Geometry: final body of the model. Coordinates: model frame, mm. A direction names the side the tool comes from. Round coordinates to 2 decimals unless told otherwise and drop trailing zeros. Loops run counter-clockwise (first coordinate to the right, second up) from the corner with the lowest first, then second, coordinate; pieces in that order, holes last. Notation, with made-up numbers: (53, 89) - (93, 89) arc R20 cw to (93, 121) - close; hole circle Ø3 at (0.25, 34.25). An arc over 180 degrees is marked (long way). Return JSON: item names as keys, results as strings. Group by question number.
1. Section A-A on x = 27. Return loops of the section in (y, z), and give its area (3 significant figures).
2. Set-up query: faces 4 (the face through (23.47, -16.04, 4.93)), 5 (the face through (-0.27, -19.57, 4.99)), 6 (the face through (0, 26, 6)), 7 (the face through (-6, -9, 10)), 8 (the face through (2.1, -7.072, 3.8)). Return all of +Z, -Z, +X, -X, +Y, -Y with unobstructed straight access to the full face (end or side cutting, diameter ignored); none if empty.
3. Draft query along Z for faces 1 (the face through (0, -12, 6)), 2 (the face through (28.79, -10.06, 4.93)), 3 (the face through (-6, -9, 0)). Return one class per face: +Z half, -Z half, draft (parallel to the pull), parting line (faces both ways), or undercut.
4. Section D-D on y = 27.5. Return loops of the section in (x, z).
5. Section C-C on z = 3. Return loops of the section in (x, y), and give its area (3 significant figures).
6. First-contact query: pin 1 Ø1 at (y, z) = (22, 3.5) entering from -X; pin 2 Ø6 at (x, z) = (0.5, 3.5) entering from -Y; pin 3 Ø1 at (x, z) = (14, 5.5) entering from -Y; pin 4 Ø2 at (x, z) = (11, 2.5) entering from +Y. Flat tips, straight axial feed; report the tip coordinate or a pass-through.
7. Material intervals for probe 1 along Z at (x, y) = (9.5, -8.5); probe 2 along Y at (x, z) = (8, 9.5); probe 3 along Y at (x, z) = (-14, 2.5), sorted ascending.
8. Section B-B on x = 0. Return loops of the section in (y, z).
from build123d import *

# Parameters (mm, degrees)
F1_DEPTH = 10
F2_DEPTH = 6
F3_DEPTH = 10
F4_START = 4
F4_DEPTH = 2


with BuildPart() as f1:
    # F0 (on Top) → F1 (new body)
    with BuildSketch(Plane.XY):
        with BuildLine():
            ThreePointArc((-28.7731093646, 19.9275732966), (0, 35), (28.7731093646, 19.9275732966))
            Line((28.7731093646, 19.9275732966), (31.0875692673, 22.4657579282))
            ThreePointArc((31.0875692673, 22.4657579282), (32.4897132735, 26.1572999971), (30.9896112585, 29.8101324057))
            ThreePointArc((30.9896112585, 29.8101324057), (-42.9603623337, 1.8458786953), (28.3184138379, -32.358421434))
            ThreePointArc((28.3184138379, -32.358421434), (31.7685286664, -27.2433524059), (32.2397786778, -21.0915114685))
            Line((32.2397786778, -21.0915114685), (32.4070255862, -17.2282779278))
            ThreePointArc((32.4070255862, -17.2282779278), (28.7073660358, -9.9847822061), (21.1130328535, -7.0724267034))
            Line((21.1130328535, -7.0724267034), (12.5, -7.0724267034))
            ThreePointArc((12.5, -7.0724267034), (0, -19.5724267034), (-12.5, -7.0724267034))
            Line((-12.5, -7.0724267034), (-17.5, -7.0724267034))
            ThreePointArc((-17.5, -7.0724267034), (-4.115416608, -24.0816402696), (15.5643824163, -15.0724267034))
            Line((15.5643824163, -15.0724267034), (21.1130328535, -15.0724267034))
            ThreePointArc((21.1130328535, -15.0724267034), (23.4950663605, -16.0636528083), (24.4707284781, -18.4521034048))
            Line((24.4707284781, -18.4521034048), (24.4390768882, -23.302781969))
            ThreePointArc((24.4390768882, -23.302781969), (24.0700935444, -24.9695381202), (23.0498717286, -26.3382500045))
            ThreePointArc((23.0498717286, -26.3382500045), (-23.3092355879, -26.108993399), (-28.7731093646, 19.9275732966))
        make_face()
    extrude(amount=F1_DEPTH)

    # F0 (on Top) → F2 (join)
    with BuildSketch(Plane.XY):
        with BuildLine():
            Line((-28.7731093646, 19.9275732966), (28.7731093646, 19.9275732966))
            ThreePointArc((28.7731093646, 19.9275732966), (0, 35), (-28.7731093646, 19.9275732966))
        make_face()
    extrude(amount=F2_DEPTH)

    # F0 (on Top) → F3 (join)
    with BuildSketch(Plane.XY):
        with BuildLine():
            ThreePointArc((-12.5, -7.0724267034), (0, -19.5724267034), (12.5, -7.0724267034))
            Line((12.5, -7.0724267034), (-12.5, -7.0724267034))
        make_face()
    extrude(amount=F3_DEPTH)

    # F0 (on Top) → F4 (cut)
    with BuildSketch(Plane.XY.offset(F4_START)):
        with BuildLine():
            ThreePointArc((-12.5, -7.0724267034), (0, -19.5724267034), (12.5, -7.0724267034))
            Line((12.5, -7.0724267034), (-12.5, -7.0724267034))
        make_face()
    extrude(amount=F4_DEPTH, mode=Mode.SUBTRACT)


solid = f1.part
Taken from the geometry:
{
 "1": {"outline": "(-33.47, 0) - (-8.72, 0) - (-8.72, 10) - (-33.47, 10) - close; (19.93, 0) - (33.47, 0) - (33.47, 10) - (22.27, 10) - (22.27, 6) - (19.93, 6) - close", "area": "374 mm2"},
 "2": {"face 4": "+Z, -Z", "face 5": "none", "face 6": "+Z", "face 7": "+Z, +X, -X, +Y, -Y", "face 8": "+Z, -Z, +X"},
 "3": {"face 1": "undercut", "face 2": "draft", "face 3": "-Z half"},
 "4": {"outline": "(-33.06, 0) - (32.3, 0) - (32.3, 10) - (21.65, 10) - (21.65, 6) - (-21.65, 6) - (-21.65, 10) - (-33.06, 10) - close"},
 "5": {"outline": "(-28.77, 19.93) - (28.77, 19.93) - (31.09, 22.47) arc R5.37 ccw to (30.99, 29.81) arc R43 ccw (long way) to (28.32, -32.36) arc R12.07 ccw to (32.24, -21.09) - (32.41, -17.23) arc R11.36 ccw to (21.11, -7.07) - (-17.5, -7.07) arc R17.5 ccw to (15.56, -15.07) - (21.11, -15.07) arc R3.36 cw to (24.47, -18.45) - (24.44, -23.3) arc R4.07 cw to (23.05, -26.34) arc R35 cw to start", "area": "2,800 mm2"},
 "6": {"pin 1": "x = -37.24", "pin 2": "y = -43", "pin 3": "y = -40.83", "pin 4": "y = 41.82"},
 "7": {"probe 1": "0 to 4, 6 to 10", "probe 2": "-42.25 to -34.07, -22.64 to -7.07, 34.07 to 42.25", "probe 3": "-40.66 to -32.08, -17.57 to -7.07, 19.93 to 40.66"},
 "8": {"outline": "(-43, 0) - (-35, 0) - (-35, 10) - (-43, 10) - close; (-24.57, 0) - (-7.07, 0) - (-7.07, 4) - (-19.57, 4) - (-19.57, 6) - (-7.07, 6) - (-7.07, 10) - (-24.57, 10) - close; (19.93, 0) - (43, 0) - (43, 10) - (35, 10) - (35, 6) - (19.93, 6) - close"}
}
